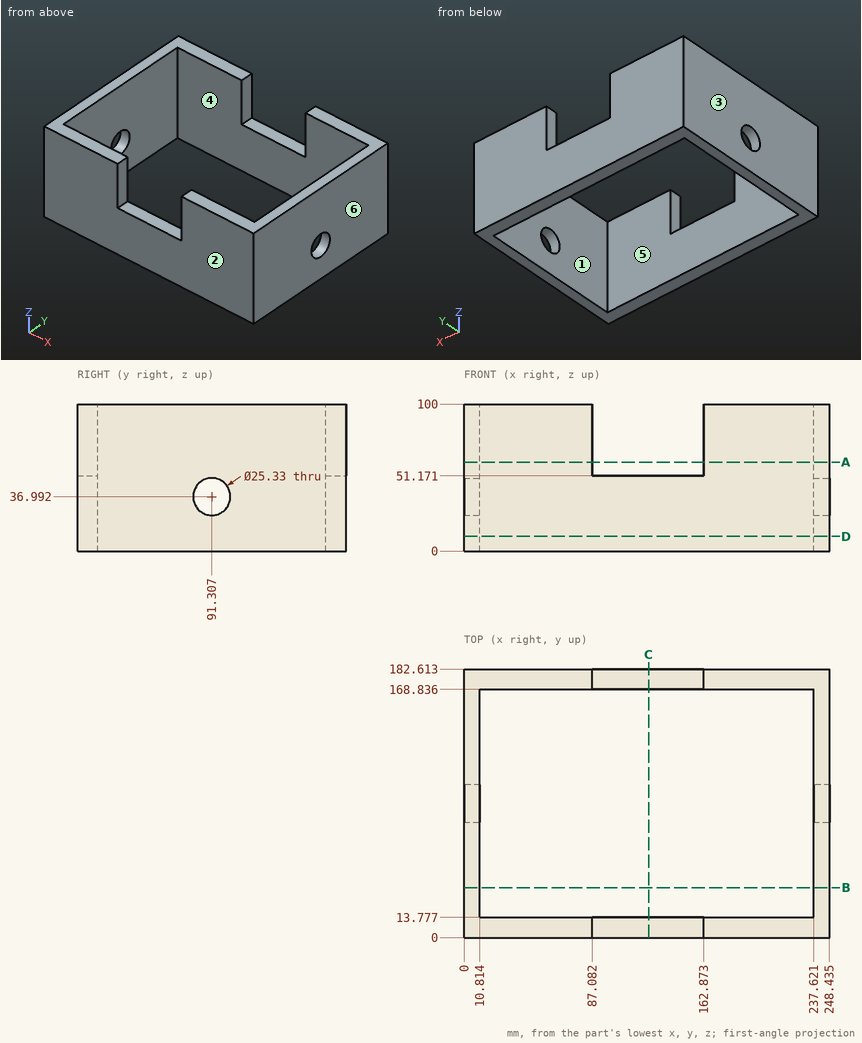
Design review of the part shown in the three views and the two pictorial views. Dimensions are in mm from the part's minimum x, y and z. A direction names the side the tool comes from. Round coordinates to 2 decimals unless told otherwise and drop trailing zeros. Write each loop counter-clockwise with the first axis right and the second up, starting at its lowest first coordinate (ties: lowest second). Pieces come first, ordered by that corner, then holes. Notation, with made-up numbers: M -4.5,-19.5 L 42.5,-19.5 A9 cw 42.5,-3.5 Z; hole C 47,-5.75 d6. An arc over 180 degrees is marked long. Use a Markdown table: item, result. Add a question column.
Q1. To check wall thickness, follow line 1 (X direction, y = 131, z = 57) (1 decimal); line 2 (Y direction, x = 52, z = 77.5). State the ranges of each line that lie inside material, in increasing order.
Q2. Insertion check: pin 1 (15 mm diameter, centred on x = 136.5, y = 4, fed in from +Z). The pin has a flat end and moves straight along its axis. Give the tip position at first contact, or say it passes through.
Q3. We need section C-C, the plane x = 125.5. State the section outline as (y, z) points, plus the area to 3 significant figures.
Q4. We need section D-D, the plane z = 10. State the section outline as (x, y) points (1 decimal), plus the area to 3 significant figures.
Q5. We need section A-A, the plane z = 60.5. State the section outline as (x, y) points (1 decimal), plus the area to 3 significant figures.
Q6. Machinability: for the marked faces 5 and 6, which of the approach directions +Z, -Z, +X, -X, +Y, -Y give a long, thin tool a straight path to every point of the face, cutting with its end or side? Answer none if there is none.
Q7. We need section B-B, the plane y = 34. State the section outline as (x, z) points (1 decimal), plus the area to 3 significant figures.
Q8. The part is to be moulded in two halves that separate along X. For the marked faces 1, 2, 3 and 4, say which applies: pulls with the +X half, pulls with the -X half, needs draft (parallel to the pull), parting line crosses it, or undercut.
Findings below:
| question | item | result |
|---|---|---|
| 1 | line 1 | x = 0 to 10.8, 237.6 to 248.4 |
| 1 | line 2 | y = 0 to 13.78, 168.84 to 182.61 |
| 2 | pin 1 | stops at z = 51.17 |
| 3 | outline | M 0,0 L 13.78,0 L 13.78,51.17 L 0,51.17 Z; M 168.84,0 L 182.61,0 L 182.61,51.17 L 168.84,51.17 Z |
| 3 | area | 1,410 mm² |
| 4 | outline | M 0,0 L 248.4,0 L 248.4,182.6 L 0,182.6 Z; hole M 10.8,13.8 L 237.6,13.8 L 237.6,168.8 L 10.8,168.8 Z |
| 4 | area | 10,200 mm² |
| 5 | outline | M 0,0 L 87.1,0 L 87.1,13.8 L 10.8,13.8 L 10.8,168.8 L 87.1,168.8 L 87.1,182.6 L 0,182.6 Z; M 162.9,0 L 248.4,0 L 248.4,182.6 L 162.9,182.6 L 162.9,168.8 L 237.6,168.8 L 237.6,13.8 L 162.9,13.8 Z |
| 5 | area | 8,110 mm² |
| 6 | face 5 | +Z, -Z |
| 6 | face 6 | +Z, -Z, +X, +Y, -Y |
| 7 | outline | M 0,0 L 10.8,0 L 10.8,100 L 0,100 Z; M 237.6,0 L 248.4,0 L 248.4,100 L 237.6,100 Z |
| 7 | area | 2,160 mm² |
| 8 | face 1 | undercut |
| 8 | face 2 | needs draft |
| 8 | face 3 | pulls with the -X half |
| 8 | face 4 | undercut |
